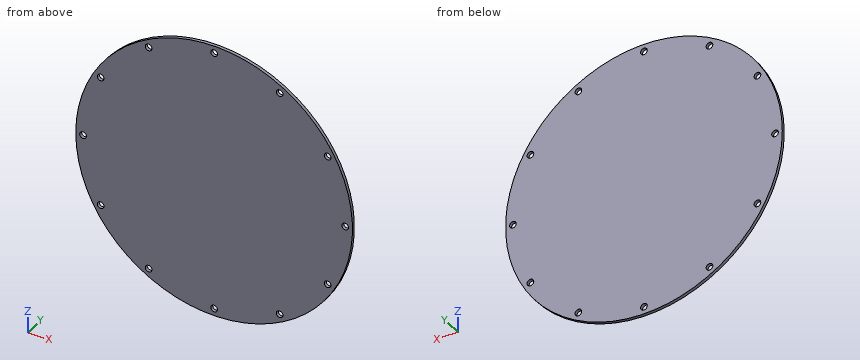
from build123d import *

# Parameters (mm, degrees)
SKETCH1_W          = 66.5
SKETCH1_H          = 1.5
SKETCH7_R          = 1.6
CUT_EXTRUDE1_DEPTH = 95.05716347
CIRPATTERN2_COUNT  = 12


with BuildPart() as part:
    # Sketch1 → Revolve1 (revolve)
    with BuildSketch(Plane.XY):
        with Locations((-33.25, 19.715)):
            Rectangle(SKETCH1_W, SKETCH1_H)
    revolve(axis=Axis((0, 20.465, 0), (0, -1, 0)))

    # Sketch7 → Cut-Extrude1 (cut, through all)
    with BuildSketch(Plane(origin=(0, 20.465, 0), x_dir=(1, 0, 0), z_dir=(0, 1, 0))):
        with Locations(Location((0, 63, 0), (0, 0, 180))):
            Circle(SKETCH7_R)
    cut_extrude1 = extrude(amount=-CUT_EXTRUDE1_DEPTH, mode=Mode.SUBTRACT)

    # CirPattern2: Cut-Extrude1 ×12 about axis
    cirpattern2_axis = Axis((0, 0, 0), (0, 1, 0))
    for i in range(1, CIRPATTERN2_COUNT):
        add(cut_extrude1.rotate(cirpattern2_axis, i * 360 / CIRPATTERN2_COUNT), mode=Mode.SUBTRACT)


solid = part.part
The listing builds one solid part. Answer for the finished solid, in the listing's coordinates (mm). Give positions to 0.01 mm unless a question says otherwise; leave off trailing zeros. Order: outer loops, then holes, each group sorted by start corner. A loop starts at its lowest first (then second) coordinate and runs counter-clockwise, first axis right, second up. Notation, with made-up numbers: (63, 81.25) - (118, 81.25) arc R24 cw to (118, 114.25) - close; hole circle Ø3 at (78.5, 53.5). An arc over 180 degrees is marked (long way). One line per item, written item: value. Start each with the question number.
1) A cutting plane is placed at A-A on z = 0. Give the vertices of the cut face in (x, y) (3 decimals), then the cut area to 3 significant figures.
2) A cutting plane is placed at C-C on x = -63. Give the vertices of the cut face in (y, z) (3 decimals), then the cut area to 3 significant figures.
3) A cutting plane is placed at B-B on z = -63. Give the vertices of the cut face in (x, y) (3 decimals), then the cut area to 3 significant figures.
4) Given pin 1 Ø1.9 at (x, z) = (-63, 0) entering from +Y; pin 2 Ø3.5 at (x, z) = (54.56, -31.5) entering from -Y (3 decimals), each flat-ended and moving along its own axis, determine where each tip first touches the part or whether it passes through.
5) A cutting plane is placed at D-D on y = 20.1. State how many separate pieces and enclosed holes the cut face has, then the cut area to 3 significant figures.
6) Find the intervals of material crossed by L1, parallel to Z at x = -0.5, y = 20.2; L2, parallel to Z at x = 55, y = 19.2; L3, parallel to X at y = 20.05, z = 26, in increasing order.
Answer sheet:
1. outline: (-66.5, 18.965) - (-64.6, 18.965) - (-64.6, 20.465) - (-66.5, 20.465) - close; (-61.4, 18.965) - (61.4, 18.965) - (61.4, 20.465) - (-61.4, 20.465) - close; (64.6, 18.965) - (66.5, 18.965) - (66.5, 20.465) - (64.6, 20.465) - close
1. area: 190 mm2
2. outline: (18.965, -21.29) - (20.465, -21.29) - (20.465, -1.6) - (18.965, -1.6) - close; (18.965, 1.6) - (20.465, 1.6) - (20.465, 21.29) - (18.965, 21.29) - close
2. area: 59.1 mm2
3. outline: (-21.29, 18.965) - (-1.6, 18.965) - (-1.6, 20.465) - (-21.29, 20.465) - close; (1.6, 18.965) - (21.29, 18.965) - (21.29, 20.465) - (1.6, 20.465) - close
3. area: 59.1 mm2
4. pin 1: passes through
4. pin 2: stops at y = 18.965
5. separate pieces: 1
5. enclosed holes: 12
5. area: 13,800 mm2
6. L1: z = -66.5 to -64.52, -61.48 to 61.48, 64.52 to 66.5
6. L2: z = -37.38 to -33.04, -29.96 to 29.96, 33.04 to 37.38
6. L3: x = -61.21 to 61.21
